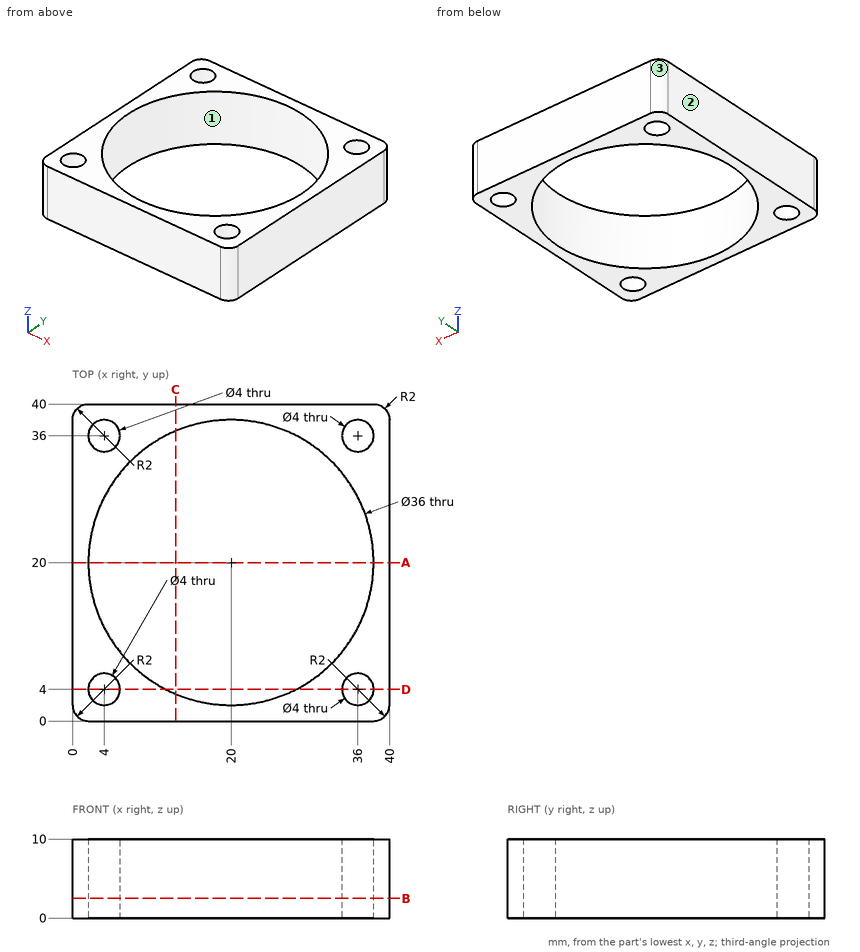
Geometry: see drawing. Coordinates: mm, zero at the bounding-box minimum. Round coordinates to 2 decimals unless told otherwise and drop trailing zeros. Loops run counter-clockwise (first coordinate to the right, second up) from the corner with the lowest first, then second, coordinate; pieces in that order, holes last. Notation, with made-up numbers: M 23,70.25 L 64,70.25 A13 ccw 64,81.25 Z; hole C 60,-16 d11. An arc over 180 degrees is marked long. Use a Markdown table: item, result. Add a question column.
1. Cut plane B-B, the plane z = 2.5. Output: boundary loops of the cut face in (x, y).
2. Cut plane C-C, the plane x = 13. Output: boundary loops of the cut face in (y, z), and give its area (3 significant figures).
3. Cut plane D-D, the plane y = 4. Output: boundary loops of the cut face in (x, z), and give its area (3 significant figures).
4. Pull-direction query (Y, two-part tool) for the marked faces 1, 2 and 3; classes: +Y half, -Y half, draft (parallel to the pull), parting line (faces both ways), or undercut.
5. Contact query for a flat-ended pin moving along its axis: pin 1 (3.5 mm diameter, centred on x = 36, y = 4, fed in from -Z). Output: stop coordinate, or through.
6. Cut plane A-A, the plane y = 20. Output: boundary loops of the cut face in (x, z), and give its area (3 significant figures).
7. Ray query, line 1 along X through (y, z) = (5, 1.5); line 2 along Y through (x, z) = (20, 4.25); line 3 along Y through (x, z) = (36, 5). Return the intervals inside material, ascending. Write a range as [from, to].
Solution:
| question | item | result |
|---|---|---|
| 1 | outline | M 0,2 A2 ccw 2,0 L 38,0 A2 ccw 40,2 L 40,38 A2 ccw 38,40 L 2,40 A2 ccw 0,38 Z; hole C 4,4 d4; hole C 20,20 d36; hole C 4,36 d4; hole C 36,4 d4; hole C 36,36 d4 |
| 2 | outline | M 0,0 L 3.42,0 L 3.42,10 L 0,10 Z; M 36.58,0 L 40,0 L 40,10 L 36.58,10 Z |
| 2 | area | 68.3 mm2 |
| 3 | outline | M 0,0 L 2,0 L 2,10 L 0,10 Z; M 6,0 L 11.75,0 L 11.75,10 L 6,10 Z; M 28.25,0 L 34,0 L 34,10 L 28.25,10 Z; M 38,0 L 40,0 L 40,10 L 38,10 Z |
| 3 | area | 155 mm2 |
| 4 | face 1 | undercut |
| 4 | face 2 | draft |
| 4 | face 3 | +Y half |
| 5 | pin 1 | passes through |
| 6 | outline | M 0,0 L 2,0 L 2,10 L 0,10 Z; M 38,0 L 40,0 L 40,10 L 38,10 Z |
| 6 | area | 40.0 mm2 |
| 7 | line 1 | x = [0, 2.27], [5.73, 10.05], [29.95, 34.27], [37.73, 40] |
| 7 | line 2 | y = [0, 2], [38, 40] |
| 7 | line 3 | y = [0, 2], [6, 11.75], [28.25, 34], [38, 40] |
